Check sheet for the modelled part. Datum: model origin and axes. Units: mm. Face numbers are marked on the shaded views. A direction names the side the tool comes from. Round coordinates to 2 decimals unless told otherwise and drop trailing zeros. Order: outer loops, then holes, each group sorted by start corner. A loop starts at its lowest first (then second) coordinate and runs counter-clockwise, first axis right, second up.
(1) Mould release check, pull along X, two halves, no side actions. Record for the marked faces 1, 2 and 3: released by +X, released by -X, zero draft, split by the parting line, or undercut.
(2) Depth check by flat-ended pin: pin 1 (4.5 mm diameter, centred on x = 89.52, z = 64.52, fed in from -Y); pin 2 (1.5 mm diameter, centred on x = -93.5, y = 30.5, fed in from -Z); pin 3 (7.5 mm diameter, centred on x = 38.77, z = -6.42, fed in from +Y). Enter the tip coordinate at first touch or a pass-through.
(3) Thickness scan on probe 1 along Y at (x, z) = (-93, -8); probe 2 along X at (y, z) = (43.5, -21); probe 3 along Z at (x, y) = (-44.5, 53). Record the ranges inside material, lowest first.
(4) Tool access check on the marked faces 4 and 5. Record the directions out of +Z, -Z, +X, -X, +Y, -Y that give a thin tool (end or side, any length) a straight path to the whole face; none if there is none.
(5) Sectioned sample at B-B, the plane z = 43. Enter the section's corners in (x, y).
(6) Sectioned sample at D-D, the plane y = 49.5. Enter the section's corners in (x, z).
(7) Sectioned sample at C-C, the plane x = -65. Enter the section's corners in (y, z), and give its area (3 significant figures).
(8) Sectioned sample at A-A, the plane z = -42. Enter the section's corners in (x, y), and give its area (3 significant figures).
```python
from build123d import *
from OCP.BRepFilletAPI import BRepFilletAPI_MakeChamfer

# Parameters (mm, degrees)
SKETCH2_W                      = 190
SKETCH2_H                      = 140
ENCLOSURE_BODY_DEPTH           = 60
FILLET1_R                      = 5
SHELL1_T                       = -3
SKETCH3_R                      = 5
SKETCH3_R_2                    = 2
SKETCH3_R_3                    = 2.85
PCB_SUPPORTS_DEPTH             = 10
ENCLOSURE_START                = 57
ENCLOSURE_CORNER_FLANGES_DEPTH = 57
SKETCH8_R                      = 3.8
CUT_EXTRUDE1_DEPTH             = 45.5
SKETCH9_R                      = 2.15
CUT_EXTRUDE2_DEPTH             = 127.472328989
CHAMFER1_SIZE                  = 2
USB_CUTOUT_DEPTH               = 6
SKETCH11_R                     = 1.6
SKETCH11_R_2                   = 6.25
SKETCH11_W                     = 12.9
SKETCH11_H                     = 19.9
BUTTON_CUTOUTS_DEPTH           = 6
CHAMFER3_SIZE                  = 1
SKETCH15_W                     = 3
SKETCH15_H                     = 12.65913529
SKETCH15_H_2                   = 57
BOSS_EXTRUDE6_DEPTH            = 10
CUT_EXTRUDE3_REACH             = 155.152
CHAMFER4_SIZE                  = 3
FILLET2_R                      = 2
BOSS_EXTRUDE7_DEPTH            = 1.5
CHAMFER5_SIZE                  = 1
CHAMFER5_SIZE2                 = 1.148564321
CHAMFER6_SIZE                  = 1
CHAMFER7_SIZE                  = 0.2
CHAMFER8_SIZE                  = 0.5


with BuildPart() as part:
    # Sketch2 → Enclosure body (new body)
    with BuildSketch(Plane(origin=(0, 0, 0), x_dir=(1, 0, 0), z_dir=(0, 1, 0))):
        Rectangle(SKETCH2_W, SKETCH2_H)
    extrude(amount=ENCLOSURE_BODY_DEPTH)

    # Fillet1
    fillet1_edges = [part.edges().sort_by_distance(p)[0] for p in [
        (95, 30, 70),
        (-95, 30, 70),
        (-95, 30, -70),
        (95, 30, -70),
    ]]
    fillet(fillet1_edges, radius=FILLET1_R)

    # Shell1
    shell1_openings = [part.faces().sort_by_distance(p)[0] for p in [
        (0, 60, 0),
    ]]
    offset(amount=SHELL1_T, openings=shell1_openings, kind=Kind.INTERSECTION)

    # Sketch3 → PCB Supports (add)
    # profile 1 of 5: a face of its own
    with BuildSketch(Plane(origin=(0, 3, 0), x_dir=(1, 0, 0), z_dir=(0, 1, 0))):
        with Locations(Location((1.270356621, 54.416611673, 0), (0, 0, 270))):
            Circle(SKETCH3_R)
        with Locations(Location((1.270356621, 54.416611673, 0), (0, 0, 270))):
            Circle(SKETCH3_R_2, mode=Mode.SUBTRACT)
    # profile 2 of 5: a face of its own
    with BuildSketch(Plane(origin=(0, 3, 0), x_dir=(1, 0, 0), z_dir=(0, 1, 0))):
        with Locations(Location((76.270356621, 54.416611673, 0), (0, 0, 270))):
            Circle(SKETCH3_R)
        with Locations(Location((76.270356621, 54.416611673, 0), (0, 0, 270))):
            Circle(SKETCH3_R_2, mode=Mode.SUBTRACT)
    # profile 3 of 5: a face of its own
    with BuildSketch(Plane(origin=(0, 3, 0), x_dir=(1, 0, 0), z_dir=(0, 1, 0))):
        with Locations(Location((76.270356621, -55.583388327, 0), (0, 0, 270))):
            Circle(SKETCH3_R)
        with Locations(Location((76.270356621, -55.583388327, 0), (0, 0, 270))):
            Circle(SKETCH3_R_2, mode=Mode.SUBTRACT)
    # profile 4 of 5: a face of its own
    with BuildSketch(Plane(origin=(0, 3, 0), x_dir=(1, 0, 0), z_dir=(0, 1, 0))):
        with Locations(Location((1.270356621, -55.583388327, 0), (0, 0, 270))):
            Circle(SKETCH3_R)
        with Locations(Location((1.270356621, -55.583388327, 0), (0, 0, 270))):
            Circle(SKETCH3_R_2, mode=Mode.SUBTRACT)
    # profile 5 of 5: a face of its own
    with BuildSketch(Plane(origin=(0, 3, 0), x_dir=(1, 0, 0), z_dir=(0, 1, 0))):
        with Locations(Location((38.770356621, 6.416611673, 0), (0, 0, 270))):
            Circle(SKETCH3_R)
        with Locations(Location((38.770356621, 6.416611673, 0), (0, 0, 270))):
            Circle(SKETCH3_R_3, mode=Mode.SUBTRACT)
    extrude(amount=PCB_SUPPORTS_DEPTH)

    # Sketch6 → Enclosure corner flanges (add)
    with BuildSketch(Plane(origin=(0, 3, 0), x_dir=(1, 0, 0), z_dir=(0, 1, 0)).offset(ENCLOSURE_START)):
        with BuildLine():
            Line((-79, 67), (-92, 54))
            Line((-92, 54), (-92, 65))
            ThreePointArc((-92, 65), (-91.414213562, 66.414213562), (-90, 67))
            Line((-90, 67), (-79, 67))
        make_face()
        with BuildLine():
            Line((-92, -54), (-79, -67))
            Line((-79, -67), (-90, -67))
            ThreePointArc((-90, -67), (-91.414213562, -66.414213562), (-92, -65))
            Line((-92, -65), (-92, -54))
        make_face()
        with BuildLine():
            Line((79, -67), (92, -54))
            Line((92, -54), (92, -65))
            ThreePointArc((92, -65), (91.414213562, -66.414213562), (90, -67))
            Line((90, -67), (79, -67))
        make_face()
        with BuildLine():
            Line((79, 67), (92, 54))
            Line((92, 54), (92, 65))
            ThreePointArc((92, 65), (91.414213562, 66.414213562), (90, 67))
            Line((90, 67), (79, 67))
        make_face()
    extrude(amount=-ENCLOSURE_CORNER_FLANGES_DEPTH)

    # Sketch8 → Cut-Extrude1 (cut)
    with BuildSketch(Plane.XZ):
        with Locations(Location((89.517766953, -64.517766953, 0), (0, 0, 270))):
            Circle(SKETCH8_R)
        with Locations(Location((89.517766953, 64.517766953, 0), (0, 0, 270))):
            Circle(SKETCH8_R)
        with Locations(Location((-89.517766953, 64.517766953, 0), (0, 0, 270))):
            Circle(SKETCH8_R)
        with Locations(Location((-89.517766953, -64.517766953, 0), (0, 0, 270))):
            Circle(SKETCH8_R)
    extrude(amount=-CUT_EXTRUDE1_DEPTH, mode=Mode.SUBTRACT)

    # Sketch9 → Cut-Extrude2 (cut, through all)
    with BuildSketch(Plane.XZ.offset(-45.5)):
        with Locations(Location((-89.517766953, 64.517766953, 0), (0, 0, 270))):
            Circle(SKETCH9_R)
        with Locations(Location((89.517766953, 64.517766953, 0), (0, 0, 270))):
            Circle(SKETCH9_R)
        with Locations(Location((89.517766953, -64.517766953, 0), (0, 0, 270))):
            Circle(SKETCH9_R)
        with Locations(Location((-89.517766953, -64.517766953, 0), (0, 0, 270))):
            Circle(SKETCH9_R)
    extrude(amount=-CUT_EXTRUDE2_DEPTH, mode=Mode.SUBTRACT)

    # Chamfer1
    chamfer1_edges = [part.edges().sort_by_distance(p)[0] for p in [
        (0, 3, 67),
        (92, 3, 0),
        (0, 3, -67),
        (-92, 3, 0),
        (-85.5, 3, 60.5),
        (85.5, 3, -60.5),
        (-85.5, 3, -60.5),
        (85.5, 3, 60.5),
    ]]
    chamfer(chamfer1_edges, length=CHAMFER1_SIZE)

    # Sketch10 → USB cutout (cut)
    with BuildSketch(Plane(origin=(95, 0, -30), x_dir=(0, 0, 1), z_dir=(-1, 0, 0))):
        with BuildLine():
            Line((29.983133645, 35), (45.983133645, 35))
            ThreePointArc((45.983133645, 35), (47.397347207, 34.414213562), (47.983133645, 33))
            Line((47.983133645, 33), (47.983133645, 26))
            ThreePointArc((47.983133645, 26), (47.397347207, 24.585786438), (45.983133645, 24))
            Line((45.983133645, 24), (29.983133645, 24))
            ThreePointArc((29.983133645, 24), (28.568920083, 24.585786438), (27.983133645, 26))
            Line((27.983133645, 26), (27.983133645, 33))
            ThreePointArc((27.983133645, 33), (28.568920083, 34.414213562), (29.983133645, 35))
        make_face()
    extrude(amount=USB_CUTOUT_DEPTH, mode=Mode.SUBTRACT)

    # Sketch11 → Button cutouts (cut)
    with BuildSketch(Plane.ZY.offset(95)):
        with Locations((-8, 39.5)):
            Circle(SKETCH11_R)
        with Locations((-8, 20.5)):
            Circle(SKETCH11_R)
        with Locations((21, 41)):
            Circle(SKETCH11_R_2)
        with Locations((21, 19)):
            Circle(SKETCH11_R_2)
        with Locations((43, 19)):
            Circle(SKETCH11_R_2)
        with Locations((43, 41)):
            Circle(SKETCH11_R_2)
        with BuildLine():
            Line((-2.121224617, 33), (-1.4, 33))
            Line((-1.4, 33), (-1.4, 27))
            Line((-1.4, 27), (-2.121224617, 27))
            ThreePointArc((-2.121224617, 27), (-14.6, 30), (-2.121224617, 33))
        make_face()
        with Locations((-41.773709578, 30)):
            Rectangle(SKETCH11_W, SKETCH11_H)
    extrude(amount=-BUTTON_CUTOUTS_DEPTH, mode=Mode.SUBTRACT)

    # Chamfer3
    chamfer3_edges = [part.edges().sort_by_distance(p)[0] for p in [
        (0, 0, 70),
        (95, 0, 0),
        (-95, 0, 0),
        (0, 0, -70),
        (93.535533906, 0, 68.535533906),
        (93.535533906, 0, -68.535533906),
        (-93.535533906, 0, -68.535533906),
        (-93.535533906, 0, 68.535533906),
    ]]
    chamfer(chamfer3_edges, length=CHAMFER3_SIZE)

    # Sketch15 → Boss-Extrude6 (add)
    with BuildSketch(Plane(origin=(-92, 0, 0), x_dir=(0, 0, -1), z_dir=(1, 0, 0))):
        with Locations((-32.569436541, 9.329567645)):
            Rectangle(SKETCH15_W, SKETCH15_H)
        with Locations((26.908015772, 31.5)):
            Rectangle(SKETCH15_W, SKETCH15_H_2)
        with Locations((-8.246855947, 31.5)):
            Rectangle(SKETCH15_W, SKETCH15_H_2)
    extrude(amount=BOSS_EXTRUDE6_DEPTH)

    # Cut-Extrude3: up to this face of the body (flat: up to its plane)
    cut_extrude3_end = Plane(part.part.faces().sort_by_distance((-86.984741784, 31.598004695, -28.408015772))[0])
    # Sketch16 → Cut-Extrude3 (cut, up to the picked face)
    with BuildSketch(Plane.XY.offset(34.069436541), mode=Mode.PRIVATE) as cut_extrude3_sk1:
        Polygon((-82, 60), (-82, 3), (-89, 60), align=None)
    cut_extrude3_tool1 = split(extrude(cut_extrude3_sk1.sketch, amount=-CUT_EXTRUDE3_REACH, mode=Mode.PRIVATE), bisect_by=cut_extrude3_end, keep=Keep.BOTH, mode=Mode.PRIVATE)
    add(cut_extrude3_tool1.solids().sort_by(Axis((-84.333333, 41, 34.069437), (0, 0, -1)))[0], mode=Mode.SUBTRACT)

    # Chamfer4
    chamfer4_edges = [part.edges().sort_by_distance(p)[0] for p in [
        (1.270356621, 3, 50.583388327),
        (76.270356621, 3, 50.583388327),
        (76.270356621, 3, -59.416611673),
        (1.270356621, 3, -59.416611673),
        (38.770356621, 3, -11.416611673),
    ]]
    chamfer(chamfer4_edges, length=CHAMFER4_SIZE)

    # Fillet2
    fillet2_edges = [part.edges().sort_by_distance(p)[0] for p in [
        (-89, 60, 8.246855947),
        (-89, 60, -26.908015772),
        (-83.55463065, 15.65913529, 32.569436541),
    ]]
    fillet(fillet2_edges, radius=FILLET2_R)

    # Sketch17 → Boss-Extrude7 (add)
    with BuildSketch(Plane(origin=(0, 60, 0), x_dir=(1, 0, 0), z_dir=(0, 1, 0))):
        Polygon((-93.5, 54.621320344), (-93.5, -54.621320344), (-79.621320344, -68.5), (79.621320344, -68.5), (93.5, -54.621320344), (93.5, 54.621320344), (79.621320344, 68.5), (-79.621320344, 68.5), align=None)
        Polygon((79, 67), (92, 54), (92, -54), (79, -67), (-79, -67), (-92, -54), (-92, 54), (-79, 67), align=None, mode=Mode.SUBTRACT)
    extrude(amount=BOSS_EXTRUDE7_DEPTH)

    # Chamfer5: one chamfer whose edges measure the first distance from different faces: ONE call of the kernel's chamfer builder (chamfer() names one face for all edges)
    chamfer5_edges_1 = [part.edges().sort_by_distance(p)[0] for p in [
        (-86, 3, 34.069436541),
        (-86, 3, 31.069436541),
        (-86, 3, -25.408015772),
        (-86, 3, -28.408015772),
        (-86, 3, 9.746855947),
        (-86, 3, 6.746855947),
    ]]
    chamfer5_edges_2 = [part.edges().sort_by_distance(p)[0] for p in [
        (-82, 3, 32.569436541),
        (-82, 3, -26.908015772),
        (-82, 3, 8.246855947),
    ]]
    chamfer5_side_2 = [part.faces().sort_by_distance(p)[0] for p in [
        (-1.487293538, 3, 0.022100072),
    ]]
    chamfer5 = BRepFilletAPI_MakeChamfer(part.part.solid().wrapped)
    for e in chamfer5_edges_1:
        chamfer5.Add(CHAMFER5_SIZE, e.wrapped)
    for e in chamfer5_edges_2:
        chamfer5.Add(CHAMFER5_SIZE, CHAMFER5_SIZE2, e.wrapped, chamfer5_side_2[0].wrapped)  # the first distance lies on this face
    add(Compound.cast(chamfer5.Shape()), mode=Mode.REPLACE)

    # Chamfer6
    chamfer6_edges = [part.edges().sort_by_distance(p)[0] for p in [
        (95, 34.414213562, 17.397347207),
        (95, 35, 7.983133645),
        (95, 34.414213562, -1.431079917),
        (95, 29.5, -2.016866355),
        (95, 24.585786438, -1.431079917),
        (95, 24, 7.983133645),
        (95, 24.585786438, 17.397347207),
        (95, 29.5, 17.983133645),
    ]]
    chamfer(chamfer6_edges, length=CHAMFER6_SIZE)

    # Chamfer7
    chamfer7_edges = [part.edges().sort_by_distance(p)[0] for p in [
        (-95, 30, -14.6),
    ]]
    chamfer(chamfer7_edges, length=CHAMFER7_SIZE)

    # Chamfer8
    chamfer8_edges = [part.edges().sort_by_distance(p)[0] for p in [
        (0, 60, 70),
        (-95, 60, 0),
        (95, 60, 0),
        (0, 60, -70),
        (93.535533906, 60, 68.535533906),
        (93.535533906, 60, -68.535533906),
        (-93.535533906, 60, -68.535533906),
        (-93.535533906, 60, 68.535533906),
    ]]
    chamfer(chamfer8_edges, length=CHAMFER8_SIZE)


solid = part.part
```
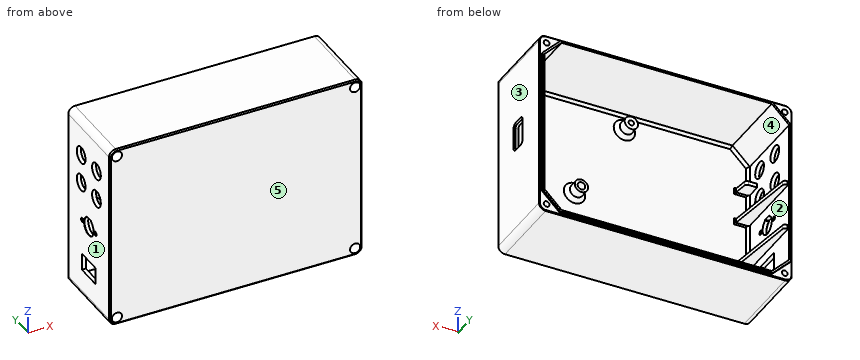
Derived:
1. face 1: released by -X
1. face 2: undercut
1. face 3: released by +X
2. pin 1: stops at y = 45.5
2. pin 2: stops at z = -69.18
2. pin 3: stops at y = 13
3. probe 1: y = 0 to 18.9, 22.1 to 23.4, 36.6 to 37.9, 41.1 to 61.5
3. probe 2: x = -95 to -92, 92 to 95
3. probe 3: z = -70 to -67, 67 to 70
4. face 4: +Y
4. face 5: +Z, -Z, +X, -X, -Y
5. outline: (-95, 1) - (-94, 0) - (94, 0) - (95, 1) - (95, 59.5) - (94.5, 60) - (93.5, 60) - (93.5, 61.5) - (92, 61.5) - (92, 5) - (90, 3) - (-90, 3) - (-92, 5) - (-92, 12.75) - (-95, 12.75) - close; (-95, 25.25) - (-92, 25.25) - (-92, 34.75) - (-95, 34.75) - close; (-95, 47.25) - (-92, 47.25) - (-92, 61.5) - (-93.5, 61.5) - (-93.5, 60) - (-94.5, 60) - (-95, 59.5) - close
6. outline: (-95, -65) arc R5 ccw to (-90, -70) - (90, -70) arc R5 ccw to (95, -65) - (95, 65) arc R5 ccw to (90, 70) - (-90, 70) arc R5 ccw to (-95, 65) - close; hole (-92, -54) - (-79, -67) - (79, -67) - (92, -54) - (92, 54) - (79, 67) - (-79, 67) - (-92, 54) - (-92, 9.75) - (-87.71, 9.75) - (-87.71, 6.75) - (-92, 6.75) - (-92, -25.41) - (-87.71, -25.41) - (-87.71, -28.41) - (-92, -28.41) - close; hole circle Ø4.3 at (-89.52, -64.52); hole circle Ø4.3 at (-89.52, 64.52); hole circle Ø4.3 at (89.52, -64.52); hole circle Ø4.3 at (89.52, 64.52)
7. outline: (0, -69) - (1, -70) - (59.5, -70) - (60, -69.5) - (60, -68.5) - (61.5, -68.5) - (61.5, -67) - (5, -67) - (3, -65) - (3, 65) - (5, 67) - (61.5, 67) - (61.5, 68.5) - (60, 68.5) - (60, 69.5) - (59.5, 70) - (1, 70) - (0, 69) - close
7. area: 769 mm2
8. outline: (-95, 1) - (-94, 0) - (94, 0) - (95, 1) - (95, 59.5) - (94.5, 60) - (93.5, 60) - (93.5, 61.5) - (92, 61.5) - (92, 5) - (90, 3) - (-90, 3) - (-92, 5) - (-92, 20.05) - (-95, 20.05) - close; (-95, 39.95) - (-92, 39.95) - (-92, 61.5) - (-93.5, 61.5) - (-93.5, 60) - (-94.5, 60) - (-95, 59.5) - close
8. area: 860 mm2
